The model under review builds one solid part; all positions refer to its coordinate system, in mm. Face numbers are marked on the shaded views. A direction names the side the tool comes from. Round coordinates to 2 decimals unless told otherwise and drop trailing zeros. Loops run counter-clockwise (first coordinate to the right, second up) from the corner with the lowest first, then second, coordinate; pieces in that order, holes last. Notation, with made-up numbers: M 3.5,-27 L 40.5,-27 A29 cw 40.5,10 Z; hole C 11.5,21.5 d11. An arc over 180 degrees is marked long. Return JSON: item names as keys, results as strings. Group by question number.
Q1. Consider section C-C (x = 6). State the section outline as (y, z) points.
Q2. Consider section D-D (y = -35). State the section outline as (x, z) points, and give its area (3 significant figures).
Q3. Consider section A-A (x = 18). State the section outline as (y, z) points, and give its area (3 significant figures).
Q4. To check wall thickness, follow line 1 along Y through (x, z) = (14, -30); line 2 along X through (y, z) = (65, -25); line 3 along X through (y, z) = (25, -28). State the ranges of each line that lie inside material, in increasing order.
Q5. Consider section B-B (y = 3). State the section outline as (x, z) points.
Q6. Draft analysis for pull direction X (two halves, no side actions). For the marked faces 1, 2, 3 and 4, state which applies: pulls with the +X half, pulls with the -X half, needs draft (parallel to the pull), parting line crosses it, or undercut.
Q7. For the marked faces 5, 6 and 7, list the 3-axis set-ups (+Z, -Z, +X, -X, +Y, -Y) from which the entire face can be reached by the end or side of a thin tool; tool diameter is ignored.
Q8. Clearance check with flat-ended pins moving along their axes: pin 1 Ø3.5 at (x, z) = (11.5, -34) entering from -Y; pin 2 Ø1.5 at (x, z) = (16.5, -34) entering from +Y; pin 3 Ø3 at (x, y) = (-14, 25) entering from -Z; pin 4 Ø8 at (x, y) = (13, 22.5) entering from -Z. State where each tip first meets the part, or that it passes through.
from build123d import *

# Parameters (mm, degrees)
BOSS_EXTRUDE1_DEPTH   = 130
SKETCH2_W             = 40
SKETCH2_H             = 10
CUT_EXTRUDE1_DEPTH    = 3
M3_TAPPED_HOLE1_D     = 2.5
M3_TAPPED_HOLE1_DEPTH = 8
M3_TAPPED_HOLE1_TIP   = 0.751075774
M3_TAPPED_HOLE2_D     = 2.5
M3_TAPPED_HOLE2_DEPTH = 8
M3_TAPPED_HOLE2_TIP   = 0.751075774
SKETCH9_W             = 52.5
SKETCH9_H             = 52.5
BOSS_EXTRUDE2_DEPTH   = 40


with BuildPart() as part:
    # Sketch1 → Boss-Extrude1 (new body)
    with BuildSketch(Plane(origin=(0, 0, 0), x_dir=(1, 0, 0), z_dir=(0, 1, 0))):
        Polygon((-20, 35), (-20, -35), (20, -35), (20, 35), (8, 35), (8, 27.5), (-8, 27.5), (-8, 35), align=None)
    extrude(amount=BOSS_EXTRUDE1_DEPTH)

    # Sketch2 → Cut-Extrude1 (cut)
    with BuildSketch(Plane(origin=(0, 0, -35), x_dir=(-1, 0, 0), z_dir=(0, 0, -1))):
        with Locations((0, 25)):
            Rectangle(SKETCH2_W, SKETCH2_H)
        with Locations((0, 65)):
            Rectangle(SKETCH2_W, SKETCH2_H)
        with Locations((0, 105)):
            Rectangle(SKETCH2_W, SKETCH2_H)
    extrude(amount=-CUT_EXTRUDE1_DEPTH, mode=Mode.SUBTRACT)

    # M3 Tapped Hole1
    with Locations(Plane(origin=(-14, 25, -32), x_dir=(-1, 0, 0), z_dir=(0, 0, -1))):
        with Locations((0, 0), (-28, 0), (0, 80), (-28, 80), (0, 40), (-28, 40)):
            Hole(M3_TAPPED_HOLE1_D / 2, depth=M3_TAPPED_HOLE1_DEPTH)
            with Locations((0, 0, -(M3_TAPPED_HOLE1_DEPTH + M3_TAPPED_HOLE1_TIP / 2))):  # 118° drill point
                Cone(0, M3_TAPPED_HOLE1_D / 2, M3_TAPPED_HOLE1_TIP, mode=Mode.SUBTRACT)

    # M3 Tapped Hole2
    with Locations(Plane(origin=(0, 25, -27.5), x_dir=(-1, 0, 0), z_dir=(0, 0, -1))):
        with Locations((0, 0), (0, 40), (0, 80)):
            Hole(M3_TAPPED_HOLE2_D / 2, depth=M3_TAPPED_HOLE2_DEPTH)
            with Locations((0, 0, -(M3_TAPPED_HOLE2_DEPTH + M3_TAPPED_HOLE2_TIP / 2))):  # 118° drill point
                Cone(0, M3_TAPPED_HOLE2_D / 2, M3_TAPPED_HOLE2_TIP, mode=Mode.SUBTRACT)

    # Sketch9 → Boss-Extrude2 (add)
    with BuildSketch(Plane.ZY.offset(20)):
        with Locations((8.75, -26.25)):
            Rectangle(SKETCH9_W, SKETCH9_H)
        with Locations((8.75, 156.25)):
            Rectangle(SKETCH9_W, SKETCH9_H)
    extrude(amount=-BOSS_EXTRUDE2_DEPTH)


solid = part.part
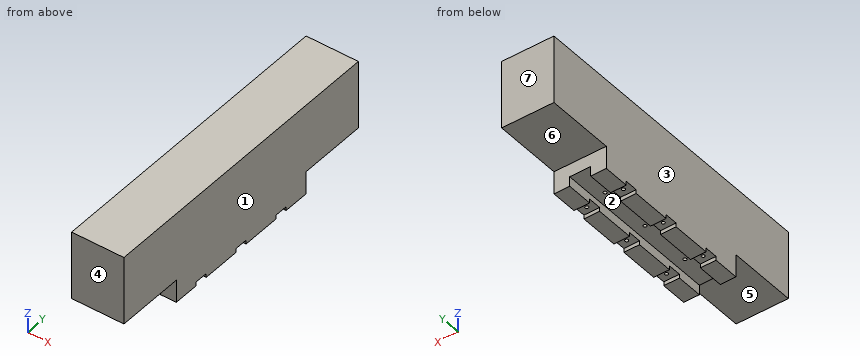
Values:
{
 "1": {"outline": "M -52.5,-17.5 L 0,-17.5 L 0,-27.5 L 130,-27.5 L 130,-17.5 L 182.5,-17.5 L 182.5,35 L -52.5,35 Z"},
 "2": {"outline": "M -20,-17.5 L 20,-17.5 L 20,35 L -20,35 Z", "area": "2,100 mm2"},
 "3": {"outline": "M -52.5,-17.5 L 0,-17.5 L 0,-35 L 20,-35 L 20,-32 L 30,-32 L 30,-35 L 60,-35 L 60,-32 L 70,-32 L 70,-35 L 100,-35 L 100,-32 L 110,-32 L 110,-35 L 130,-35 L 130,-17.5 L 182.5,-17.5 L 182.5,35 L -52.5,35 Z", "area": "14,500 mm2"},
 "4": {"line 1": "y = 0 to 23.75, 26.25 to 63.75, 66.25 to 103.75, 106.25 to 130", "line 2": "x = -20 to -15.25, -12.75 to -1.25, 1.25 to 12.75, 15.25 to 20", "line 3": "x = -20 to -15.25, -12.75 to -8, 8 to 12.75, 15.25 to 20"},
 "5": {"outline": "M -20,-35 L -8,-35 L -8,-27.5 L 8,-27.5 L 8,-35 L 20,-35 L 20,35 L -20,35 Z"},
 "6": {"face 1": "pulls with the +X half", "face 2": "undercut", "face 3": "pulls with the -X half", "face 4": "needs draft"},
 "7": {"face 5": "-Z, +X, -X, -Y", "face 6": "-Z, +X, -X, +Y", "face 7": "+Z, -Z, +X, -X, +Y"},
 "8": {"pin 1": "stops at y = 0", "pin 2": "stops at y = 130", "pin 3": "stops at z = -32", "pin 4": "stops at z = -35"}
}
